Here's how the part is built. I have some questions about the finished solid (model axes, mm). Coordinates: 2 decimals unless noted, no trailing zeros. Write each loop counter-clockwise with the first axis right and the second up, starting at its lowest first coordinate (ties: lowest second). Pieces come first, ordered by that corner, then holes. Notation, with made-up numbers: M 0.25,4.25 L 8.25,4.25 A17 ccw 8.25,19.25 Z; hole C 81.25,28.25 d3. An arc over 180 degrees is marked long. Write each question's results on one line, items separated by ' | '. Start each with the question number.
from build123d import *

# Parameters (mm, degrees)
SKETCH1_3_R         = 1.5
SKETCH1_3_R_2       = 4
SKETCH1_3_R_3       = 2
BOSS_EXTRUDE2_DEPTH = 1.25
FILLET2_R           = 10


with BuildPart() as part:
    # Sketch1_3 → Boss-Extrude2 (new, symmetric)
    with BuildSketch(Plane.XY):
        Polygon((50, 37.5), (-50, 37.5), (-50, -12.5), (-25, -37.5), (25, -37.5), (50, -12.5), align=None)
        with Locations((0, -29.5)):
            Circle(SKETCH1_3_R, mode=Mode.SUBTRACT)
        with Locations((-16.5, -27.75)):
            Circle(SKETCH1_3_R, mode=Mode.SUBTRACT)
        with Locations((16.5, -27.75)):
            Circle(SKETCH1_3_R, mode=Mode.SUBTRACT)
        with Locations((-38.5, 17.5)):
            Circle(SKETCH1_3_R_2, mode=Mode.SUBTRACT)
        with Locations((38.5, 17.5)):
            Circle(SKETCH1_3_R_2, mode=Mode.SUBTRACT)
        with Locations((-16.5, -2.75)):
            Circle(SKETCH1_3_R_3, mode=Mode.SUBTRACT)
        with Locations((16.5, -2.75)):
            Circle(SKETCH1_3_R_3, mode=Mode.SUBTRACT)
        with Locations((38.5, 27.5)):
            Circle(SKETCH1_3_R, mode=Mode.SUBTRACT)
        with Locations((-38.5, 27.5)):
            Circle(SKETCH1_3_R, mode=Mode.SUBTRACT)
        with Locations((0, 12.5)):
            Circle(SKETCH1_3_R, mode=Mode.SUBTRACT)
        with Locations((0, 27.5)):
            Circle(SKETCH1_3_R, mode=Mode.SUBTRACT)
    extrude(amount=BOSS_EXTRUDE2_DEPTH, both=True)

    # Fillet2
    fillet2_edges = [part.edges().sort_by_distance(p)[0] for p in [
        (50, -12.5, 0),
        (25, -37.5, 0),
        (-25, -37.5, 0),
        (-50, -12.5, 0),
        (-50, 37.5, 0),
        (50, 37.5, 0),
    ]]
    fillet(fillet2_edges, radius=FILLET2_R)


solid = part.part
1) I want a section at D-D, the plane x = -16.5. Write out the boundary of the cut face in (y, z), then the cut area to 3 significant figures.
2) I want a section at B-B, the plane x = 0. Write out the boundary of the cut face in (y, z), then the cut area to 3 significant figures.
3) For pin 1 Ø1.8 at (x, y) = (-16.5, -27.75) entering from +Z; pin 2 Ø1 at (x, z) = (-27, 0) entering from -Y; pin 3 Ø1 at (y, z) = (-15.5, 1) entering from +X, each with a flat end and sliding along its axis, tell me the tip position at first contact or that it passes through.
4) Please list where these lines run through material, in increasing order: line 1 (Y direction, x = -16.5, z = 0.1); line 2 (X direction, y = -4.5, z = 0.85); line 3 (Y direction, x = -38.5, z = -0.5). Write a range as [from, to].
5) I want a section at C-C, the plane z = -0.4. Give the number of separate pieces and of enclosed holes in the cut face, then the cut area to 3 significant figures.
6) We'd pull the mould along X, two halves only. Please class faces 1 (the cylindrical face through (-18.087, -3.967, -0.018)), 2 (the flat face through (-37.6, -24.9, 0)), 3 (the flat face through (1, 37.5, 0)): pulls with the +X half, pulls with the -X half, needs draft (parallel to the pull), parting line crosses it, or undercut.
7) I want a section at A-A, the plane y = 17.5. Write out the boundary of the cut face in (x, z), then the cut area to 3 significant figures.
Output:
1) outline: M -37.5,-1.25 L -29.25,-1.25 L -29.25,1.25 L -37.5,1.25 Z; M -26.25,-1.25 L -4.75,-1.25 L -4.75,1.25 L -26.25,1.25 Z; M -0.75,-1.25 L 37.5,-1.25 L 37.5,1.25 L -0.75,1.25 Z | area: 170 mm2
2) outline: M -37.5,-1.25 L -31,-1.25 L -31,1.25 L -37.5,1.25 Z; M -28,-1.25 L 11,-1.25 L 11,1.25 L -28,1.25 Z; M 14,-1.25 L 26,-1.25 L 26,1.25 L 14,1.25 Z; M 29,-1.25 L 37.5,-1.25 L 37.5,1.25 L 29,1.25 Z | area: 165 mm2
3) pin 1: passes through | pin 2: stops at y = -35.76 | pin 3: stops at x = 47.48
4) line 1: y = [-37.5, -29.25], [-26.25, -4.75], [-0.75, 37.5] | line 2: x = [-50, -17.47], [-15.53, 15.53], [17.47, 50] | line 3: y = [-24, 13.5], [21.5, 26], [29, 37.5]
5) separate pieces: 1 | enclosed holes: 11 | area: 6,650 mm2
6) face 1: undercut | face 2: pulls with the -X half | face 3: needs draft
7) outline: M -50,-1.25 L -42.5,-1.25 L -42.5,1.25 L -50,1.25 Z; M -34.5,-1.25 L 34.5,-1.25 L 34.5,1.25 L -34.5,1.25 Z; M 42.5,-1.25 L 50,-1.25 L 50,1.25 L 42.5,1.25 Z | area: 210 mm2
